Can you work these out from the model? Positions are in its coordinate system, mm. Round coordinates to 2 decimals unless told otherwise and drop trailing zeros. Order: outer loops, then holes, each group sorted by start corner. A loop starts at its lowest first (then second) coordinate and runs counter-clockwise, first axis right, second up.
Q1. If we section it at B-B (y = 3): Count the separate pieces of the cut face and the enclosed holes in it, plus the area to 3 significant figures.
Q2. If we section it at A-A (z = 267.5): Please give me the cut outline in (x, y) (3 decimals), plus the area to 3 significant figures.
Q3. If I drill on line 1 (Z direction, x = -46, y = 5.5); line 2 (X direction, y = 2, z = 179.5) (3 decimals); line 3 (X direction, y = 0.75, z = 340.5) (3 decimals), over which ranges is the centre line in solid material (lowest first)?
from build123d import *

# Parameters (mm, degrees)
SKETCH1_W           = 914.4
SKETCH1_H           = 1219.2
BOSS_EXTRUDE1_DEPTH = 6.35
SKETCH2_R           = 3.2639
CUT_EXTRUDE1_DEPTH  = 763.026457874
SKETCH3_R           = 2.5908
SKETCH3_W           = 567.7408
SKETCH3_H           = 565.15
CUT_EXTRUDE2_DEPTH  = 763.026457874


with BuildPart() as part:
    # Sketch1 → Boss-Extrude1 (new body)
    with BuildSketch(Plane(origin=(0, 0, 0), x_dir=(1, 0, 0), z_dir=(0, 1, 0))):
        Rectangle(SKETCH1_W, SKETCH1_H)
    extrude(amount=BOSS_EXTRUDE1_DEPTH)

    # Sketch2 → Cut-Extrude1 (cut, through all)
    with BuildSketch(Plane.XZ):
        with Locations(Location((56.9595, 498.8814, 0), (0, 0, 270))):
            Circle(SKETCH2_R)
        with Locations(Location((82.3595, 498.8814, 0), (0, 0, 270))):
            Circle(SKETCH2_R)
        with Locations(Location((446.0875, 498.8814, 0), (0, 0, 270))):
            Circle(SKETCH2_R)
        with Locations(Location((420.6875, 498.8814, 0), (0, 0, 270))):
            Circle(SKETCH2_R)
        with Locations(Location((61.722, -498.8814, 0), (0, 0, 270))):
            Circle(SKETCH2_R)
        with Locations(Location((87.122, -498.8814, 0), (0, 0, 270))):
            Circle(SKETCH2_R)
        with Locations(Location((420.878, -498.8814, 0), (0, 0, 270))):
            Circle(SKETCH2_R)
        with Locations(Location((446.278, -498.8814, 0), (0, 0, 270))):
            Circle(SKETCH2_R)
    extrude(amount=-CUT_EXTRUDE1_DEPTH, mode=Mode.SUBTRACT)

    # Sketch3 → Cut-Extrude2 (cut, through all)
    with BuildSketch(Plane(origin=(0, 6.35, 0), x_dir=(1, 0, 0), z_dir=(0, 1, 0))):
        with Locations(Location((241.3, 171.704, 0), (0, 0, 270))):
            Circle(SKETCH3_R)
        with Locations(Location((241.3, 54.864, 0), (0, 0, 270))):
            Circle(SKETCH3_R)
        with Locations(Location((241.3, -61.976, 0), (0, 0, 270))):
            Circle(SKETCH3_R)
        with Locations(Location((241.3, -178.816, 0), (0, 0, 270))):
            Circle(SKETCH3_R)
        with Locations(Location((241.3, -295.656, 0), (0, 0, 270))):
            Circle(SKETCH3_R)
        with Locations(Location((241.3, -412.496, 0), (0, 0, 270))):
            Circle(SKETCH3_R)
        with Locations(Location((-342.9, -412.496, 0), (0, 0, 270))):
            Circle(SKETCH3_R)
        with Locations(Location((-226.06, -412.496, 0), (0, 0, 270))):
            Circle(SKETCH3_R)
        with Locations(Location((-109.22, -412.496, 0), (0, 0, 270))):
            Circle(SKETCH3_R)
        with Locations(Location((7.62, -412.496, 0), (0, 0, 270))):
            Circle(SKETCH3_R)
        with Locations(Location((124.46, -412.496, 0), (0, 0, 270))):
            Circle(SKETCH3_R)
        with Locations(Location((-342.9, -295.656, 0), (0, 0, 270))):
            Circle(SKETCH3_R)
        with Locations(Location((-342.9, -178.816, 0), (0, 0, 270))):
            Circle(SKETCH3_R)
        with Locations(Location((-342.9, -61.976, 0), (0, 0, 270))):
            Circle(SKETCH3_R)
        with Locations(Location((-342.9, 54.864, 0), (0, 0, 270))):
            Circle(SKETCH3_R)
        with Locations(Location((124.46, 171.704, 0), (0, 0, 270))):
            Circle(SKETCH3_R)
        with Locations(Location((7.62, 171.704, 0), (0, 0, 270))):
            Circle(SKETCH3_R)
        with Locations(Location((-109.22, 171.704, 0), (0, 0, 270))):
            Circle(SKETCH3_R)
        with Locations(Location((-226.06, 171.704, 0), (0, 0, 270))):
            Circle(SKETCH3_R)
        with Locations(Location((-342.9, 171.704, 0), (0, 0, 270))):
            Circle(SKETCH3_R)
        with Locations((-49.5046, -120.396)):
            Rectangle(SKETCH3_W, SKETCH3_H)
    extrude(amount=-CUT_EXTRUDE2_DEPTH, mode=Mode.SUBTRACT)


solid = part.part
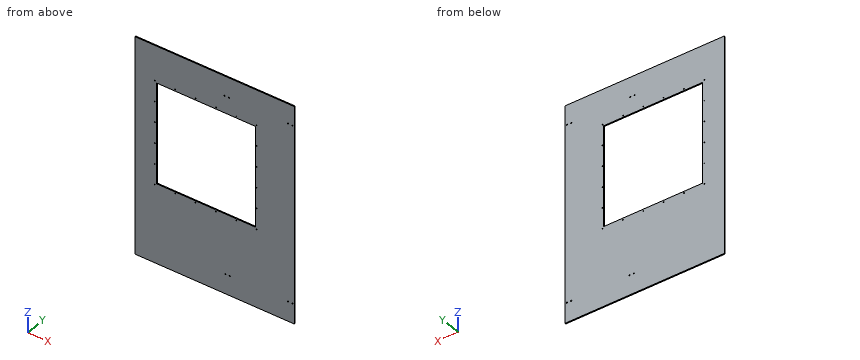
Solution:
1. separate pieces: 1
1. enclosed holes: 29
1. area: 793,000 mm2
2. outline: (-457.2, 0) - (-333.375, 0) - (-333.375, 6.35) - (-457.2, 6.35) - close; (234.366, 0) - (457.2, 0) - (457.2, 6.35) - (234.366, 6.35) - close
2. area: 2,200 mm2
3. line 1: z = -609.6 to -162.18, 402.97 to 609.6
3. line 2: x = -457.2 to -345.399, -340.401 to -333.375, 234.366 to 238.801, 243.799 to 457.2
3. line 3: x = -457.2 to -333.375, 234.366 to 457.2
